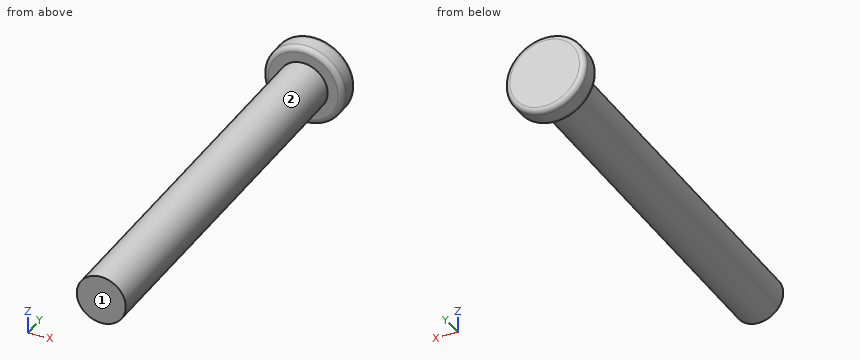
from build123d import *

# Parameters (mm, degrees)
SKETCH1_R           = 1.2065
BOSS_EXTRUDE1_DEPTH = 19.05
SKETCH2_R           = 1.9685
BOSS_EXTRUDE2_DEPTH = 1.143
FILLET1_R           = 0.254


with BuildPart() as part:
    # Sketch1 → Boss-Extrude1 (new body)
    with BuildSketch(Plane(origin=(0, 0, 0), x_dir=(1, 0, 0), z_dir=(0, 1, 0))):
        with Locations(Location((0, 0, 0), (0, 0, 90))):
            Circle(SKETCH1_R)
    extrude(amount=BOSS_EXTRUDE1_DEPTH)

    # Sketch2 → Boss-Extrude2 (add)
    with BuildSketch(Plane(origin=(0, 19.05, 0), x_dir=(1, 0, 0), z_dir=(0, 1, 0))):
        with Locations(Location((0, 0, 0), (0, 0, 270))):
            Circle(SKETCH2_R)
    extrude(amount=BOSS_EXTRUDE2_DEPTH)

    # Fillet1
    fillet1_edges = [part.edges().sort_by_distance(p)[0] for p in [
        (0, 19.05, -1.9685),
        (0, 20.193, -1.9685),
    ]]
    fillet(fillet1_edges, radius=FILLET1_R)


solid = part.part
Could you check a few things on this model? Use its own coordinates, in mm. Face numbers are marked on the shaded views. A direction names the side the tool comes from. Give positions to 0.01 mm unless a question says otherwise; leave off trailing zeros. Write each loop counter-clockwise with the first axis right and the second up, starting at its lowest first coordinate (ties: lowest second). Pieces come first, ordered by that corner, then holes. Notation, with made-up numbers: (75, 83) -> (82, 83) arc R8 ccw to (82, 90) -> close; hole circle Ø1 at (48.5, 57). An arc over 180 degrees is marked (long way). Write each question's results on one line, items separated by ' | '. Start each with the question number.
Q1. Which directions (+Z, -Z, +X, -X, +Y, -Y) give clear straight access to the entire face, cutting with the end or side of a thin tool? Please do the marked faces 1 and 2.
Q2. Suppose I cut it at B-B, the plane z = 0. List the corners of the cut face in (x, y) for me.
Q3. Suppose I cut it at C-C, the plane y = 3.5. List the corners of the cut face in (x, z) for me, and give its area (3 significant figures).
Q4. I need wall thicknesses on probe 1 along Y at (x, z) = (-0.85, -1.3); probe 2 along Z at (x, y) = (0.3, 9.5). Which ranges of each line are inside material? Lowest first, please.
Q5. Suppose I cut it at A-A, the plane x = 0. List the corners of the cut face in (y, z) for me.
Outcome:
1) face 1: +Z, -Z, +X, -X, -Y | face 2: -Y
2) outline: (-1.97, 19.3) arc R0.25 ccw to (-1.71, 19.05) -> (-1.21, 19.05) -> (-1.21, 0) -> (1.21, 0) -> (1.21, 19.05) -> (1.71, 19.05) arc R0.25 ccw to (1.97, 19.3) -> (1.97, 19.94) arc R0.25 ccw to (1.71, 20.19) -> (-1.71, 20.19) arc R0.25 ccw to (-1.97, 19.94) -> close
3) outline: circle Ø2.41 at (0, 0) | area: 4.57 mm2
4) probe 1: 19.05 to 20.19 | probe 2: -1.17 to 1.17
5) outline: (0, -1.21) -> (19.05, -1.21) -> (19.05, -1.71) arc R0.25 ccw to (19.3, -1.97) -> (19.94, -1.97) arc R0.25 ccw to (20.19, -1.71) -> (20.19, 1.71) arc R0.25 ccw to (19.94, 1.97) -> (19.3, 1.97) arc R0.25 ccw to (19.05, 1.71) -> (19.05, 1.21) -> (0, 1.21) -> close
